Model file for the job. Use its own axes, mm. A direction names the side the tool comes from. Round coordinates to 2 decimals unless told otherwise and drop trailing zeros. Loops run counter-clockwise (first coordinate to the right, second up) from the corner with the lowest first, then second, coordinate; pieces in that order, holes last. Notation, with made-up numbers: M 31,26.5 L 72,26.5 A15 ccw 72,33.5 Z; hole C 16.25,-12.5 d11. An arc over 180 degrees is marked long. Use a Markdown table: item, result. Add a question column.
Item 1: Saw through at A-A on z = 9. Write the cut outline in (x, y).
Item 2: Tool access for faces 1 (the flat face through (8.788, 324, 6)), 2 (the flat face through (11.963, 32, 6)), 3 (the flat face through (7.73, 176, 6)): list every direction of +Z, -Z, +X, -X, +Y, -Y with a clear straight run to the whole face (end or side of a thin tool).
Item 3: Wall check: L1, parallel to X at y = 28.5, z = 6; L2, parallel to X at y = 281, z = 3; L3, parallel to Y at x = 9.5, z = 4. Give the ranges that are in metal, low to high. Write a range as from..to.
Item 4: Two-plate mould, pull along X, no slides. Class faces 4 (the flat face through (9.877, 32, 6)), 5 (the flat face through (25.4, 175, 16)), 6 (the flat face through (13, 355.6, 16)): +X half, -X half, draft (parallel to the pull), parting line (faces both ways), or undercut.
Item 5: Saw through at C-C on y = 26. Write the cut outline in (x, z), then the cut area to 3 significant figures.
Item 6: Saw through at B-B on y = 316. Write the cut outline in (x, z).
```python
from build123d import *

# Parameters (mm, degrees)
F1_DEPTH = 25.4
F2_W     = 3.175
F2_H     = 63.5
F2_W_2   = 2.085983
F3_DEPTH = 12.7
F4_W     = 355.6
F4_H     = 58.603869
F5_DEPTH = 25.4


with BuildPart() as f1:
    # F0 (on Right) → F1 (new body)
    with BuildSketch(Plane.YZ):
        with BuildLine():
            Line((0, 19.445715), (0, 0))
            Line((0, 0), (355.6, 0))
            Line((355.6, 0), (355.6, 19.445715))
            Line((355.6, 19.445715), (355.6, 31.75))
            Line((355.6, 31.75), (343.690661, 32.121079))
            ThreePointArc((343.690661, 32.121079), (300.578253, 39.833745), (260.35, 57.15))
            ThreePointArc((260.35, 57.15), (177.8, 76.307596), (95.25, 57.15))
            ThreePointArc((95.25, 57.15), (55.021747, 39.833745), (11.909339, 32.121079))
            Line((11.909339, 32.121079), (0, 31.75))
            Line((0, 31.75), (0, 19.445715))
        make_face()
    extrude(amount=F1_DEPTH)

    # F2 (on face) → F3 (cut)
    with BuildSketch(Plane(origin=(0, 0, 0), x_dir=(1, 0, 0), z_dir=(0, 0, -1))):
        Polygon((11.9634, -292.1), (11.9634, -63.5), (9.877417, -63.5), (7.730067, -63.5), (7.730067, -292.1), (8.7884, -292.1), align=None)
        with Locations((10.3759, -323.85)):
            Rectangle(F2_W, F2_H)
        with Locations((10.920409, -31.75)):
            Rectangle(F2_W_2, F2_H)
    extrude(amount=-F3_DEPTH, mode=Mode.SUBTRACT)

    # F4 (on face) → F5 (cut)
    with BuildSketch(Plane.YZ.offset(25.4)):
        with Locations((177.8, 61.051934)):
            Rectangle(F4_W, F4_H)
    extrude(amount=-F5_DEPTH, mode=Mode.SUBTRACT)


solid = f1.part
```
Entries:
| question | item | result |
|---|---|---|
| 1 | outline | M 0,0 L 9.88,0 L 9.88,63.5 L 7.73,63.5 L 7.73,292.1 L 8.79,292.1 L 8.79,355.6 L 0,355.6 Z; M 11.96,0 L 25.4,0 L 25.4,355.6 L 11.96,355.6 Z |
| 2 | face 1 | -Z, +Y |
| 2 | face 2 | -Z, +Y, -Y |
| 2 | face 3 | -Z |
| 3 | L1 | 0..9.88, 11.96..25.4 |
| 3 | L2 | 0..7.73, 11.96..25.4 |
| 3 | L3 | 0..63.5 |
| 4 | face 4 | undercut |
| 4 | face 5 | +X half |
| 4 | face 6 | draft |
| 5 | outline | M 0,0 L 9.88,0 L 9.88,12.7 L 11.96,12.7 L 11.96,0 L 25.4,0 L 25.4,31.75 L 0,31.75 Z |
| 5 | area | 780 mm2 |
| 6 | outline | M 0,0 L 8.79,0 L 8.79,12.7 L 11.96,12.7 L 11.96,0 L 25.4,0 L 25.4,31.75 L 0,31.75 Z |
